The model under review builds one solid part; all positions refer to its coordinate system, in mm. A direction names the side the tool comes from. Coordinates: 2 decimals unless noted, no trailing zeros. Write each loop counter-clockwise with the first axis right and the second up, starting at its lowest first coordinate (ties: lowest second). Pieces come first, ordered by that corner, then holes.
```python
from build123d import *

# Parameters (mm, degrees)
CORPS_VERROU_GUILLOTINE_START         = -4.5
CORPS_VERROU_GUILLOTINE_DEPTH         = 5
LUMIERE_OBLONGUE_MANIVELLE_DEPTH      = 43.231504828
LUMIERE_OBLONGUE_MANIVELLE_DEPTH_BACK = 43.231504828


with BuildPart() as part:
    # Esquisse1 → Corps_verrou_guillotine (new body)
    with BuildSketch(Plane.XY.offset(CORPS_VERROU_GUILLOTINE_START)):
        Polygon((-19, 36.5), (19, 36.5), (19, 28.5), (14, 28.5), (14, 2.5), (-14, 2.5), (-14, 28.5), (-19, 28.5), align=None)
    extrude(amount=-CORPS_VERROU_GUILLOTINE_DEPTH)

    # Esquisse2 → Lumiere_oblongue_manivelle (cut, two sides: drawn at the far end of the back side and taken through both)
    with BuildSketch(Plane.XY.offset(-LUMIERE_OBLONGUE_MANIVELLE_DEPTH_BACK)):
        with BuildLine():
            Line((-11.5, 34.5), (11.5, 34.5))
            ThreePointArc((11.5, 34.5), (13.5, 32.5), (11.5, 30.5))
            Line((11.5, 30.5), (-11.5, 30.5))
            ThreePointArc((-11.5, 30.5), (-13.5, 32.5), (-11.5, 34.5))
        make_face()
    extrude(amount=LUMIERE_OBLONGUE_MANIVELLE_DEPTH + LUMIERE_OBLONGUE_MANIVELLE_DEPTH_BACK, mode=Mode.SUBTRACT)


solid = part.part
```
Item 1: Take a section at C-C, the plane z = -5.55. Write out the cut boundary in (x, y), plus the area to 3 significant figures.
Solved:
outline: (-19, 28.5) - (-14, 28.5) - (-14, 2.5) - (14, 2.5) - (14, 28.5) - (19, 28.5) - (19, 36.5) - (-19, 36.5) - close; hole (-11.5, 30.5) - (11.5, 30.5) arc R2 ccw to (11.5, 34.5) - (-11.5, 34.5) arc R2 ccw to start
area: 927 mm2
Item 2: Machinability: for faces 4 (the face through (17, 28.5, -7)), 5 (the face through (0, 20, -9.5)), 6 (the face through (0, 30.5, -7)), 7 (the face through (0, 20, -4.5)), 8 (the face through (-16, 28.5, -7)), which of the approach directions +Z, -Z, +X, -X, +Y, -Y give a long, thin tool a straight path to every point of the face, cutting with its end or side? Answer none if there is none.
Solved:
face 4: +Z, -Z, +X, -Y
face 5: -Z, +X, -X, +Y, -Y
face 6: +Z, -Z
face 7: +Z, +X, -X, +Y, -Y
face 8: +Z, -Z, -X, -Y
Item 3: Take a section at B-B, the plane y = 32.5. Write out the cut boundary in (x, z), plus the area to 3 significant figures.
Solved:
outline: (-19, -9.5) - (-13.5, -9.5) - (-13.5, -4.5) - (-19, -4.5) - close; (13.5, -9.5) - (19, -9.5) - (19, -4.5) - (13.5, -4.5) - close
area: 55.0 mm2
Item 4: Mouldability with a two-part tool opening along X and no side actions: class faces 1 (the face through (-13.5, 32.5, -7)), 2 (the face through (19, 33, -7)), 3 (the face through (-14, 15, -7)) as pulls with the +X half, pulls with the -X half, needs draft (parallel to the pull), parting line crosses it, or undercut.
Solved:
face 1: undercut
face 2: pulls with the +X half
face 3: pulls with the -X half
Item 5: For pin 1 (1.5 mm diameter, centred on x = 15.5, z = -6, fed in from -Y); pin 2 (1.5 mm diameter, centred on y = 15.5, z = -8, fed in from +X), all flat-tipped, find the tip position at first contact; note any pin that passes through.
Solved:
pin 1: stops at y = 28.5
pin 2: stops at x = 14
Item 6: To check wall thickness, follow line 1 along Y through (x, z) = (-4, -6.6); line 2 along X through (y, z) = (6.5, -6.5); line 3 along Y through (x, z) = (-12, -7.2). State the ranges of each line that lie inside material, in increasing order.
Solved:
line 1: y = 2.5 to 30.5, 34.5 to 36.5
line 2: x = -14 to 14
line 3: y = 2.5 to 30.56, 34.44 to 36.5
Item 7: Take a section at A-A, the plane x = 6.5. Write out the cut boundary in (y, z).
Solved:
outline: (2.5, -9.5) - (30.5, -9.5) - (30.5, -4.5) - (2.5, -4.5) - close; (34.5, -9.5) - (36.5, -9.5) - (36.5, -4.5) - (34.5, -4.5) - close
Item 8: Take a section at D-D, the plane y = 17.5. Write out the cut boundary in (x, z), plus the area to 3 significant figures.
Solved:
outline: (-14, -9.5) - (14, -9.5) - (14, -4.5) - (-14, -4.5) - close
area: 140 mm2
